from build123d import *

# Parameters (mm, degrees)
CUT_EXTRUDE_1_DEPTH = 0.495


with BuildPart() as part:
    # 草图1 → 旋转1 (revolve)
    with BuildSketch(Plane.XY, mode=Mode.PRIVATE) as revolve_1_sk:
        with BuildLine():
            Line((0, 0), (2.75, 0))
            Line((2.75, 0), (1.747011561, 1.038624933))
            ThreePointArc((1.747011561, 1.038624933), (1.564086143, 1.320305375), (1.5, 1.65))
            Line((1.5, 1.65), (1.5, 10))
            Line((1.5, 10), (0, 10))
            Line((0, 10), (0, 0))
        make_face()
    revolve(revolve_1_sk.sketch.rotate(Axis((0, 3.09547163, 0), (0, -1, 0)), 90), axis=Axis((0, 3.09547163, 0), (0, -1, 0)))

    # 草图2 → 切除-拉伸1 (cut)
    with BuildSketch(Plane.XZ):
        Polygon((-0.375, -0.375), (-0.375, -1.925), (0.375, -1.925), (0.375, -0.375), (1.925, -0.375), (1.925, 0.375), (0.375, 0.375), (0.375, 1.925), (-0.375, 1.925), (-0.375, 0.375), (-1.925, 0.375), (-1.925, -0.375), align=None)
    extrude(amount=-CUT_EXTRUDE_1_DEPTH, mode=Mode.SUBTRACT)


solid = part.part
For this review, take the finished solid that the model builds, in its own axes (mm). Round coordinates to 2 decimals unless told otherwise and drop trailing zeros. Order: outer loops, then holes, each group sorted by start corner. A loop starts at its lowest first (then second) coordinate and runs counter-clockwise, first axis right, second up. Notation, with made-up numbers: M 31,67 L 49,67 A29 cw 49,100 Z; hole C -2.75,39 d7. An arc over 180 degrees is marked long. Write each question's results on one line, items separated by ' | '. Start each with the question number.
1. Add section B-B (x = 0). State the section outline as (y, z) points (3 decimals), then the cut area to 3 significant figures.
2. Add section C-C (y = 7.5). State the section outline as (x, z) points, then the cut area to 3 significant figures.
3. Clearance check with flat-ended pins moving along their axes: pin 1 Ø3 at (x, y) = (0, 8.5) entering from -Z; pin 2 Ø0.5 at (y, z) = (0, -1.5) entering from +X. State where each tip first meets the part, or that it passes through.
4. To check wall thickness, follow L1, parallel to Y at x = 1.45, z = -0.15 (3 decimals); L2, parallel to X at y = 6.75, z = -0.15; L3, parallel to X at y = 5, z = -1.3. State the ranges of each line that lie inside material, in increasing order. Write a range as [from, to].
5. Draft analysis for pull direction X (two halves, no side actions). For faces 1 (the face through (-0.45, 5.88, 1.43)), 2 (the face through (0, 0.495, 0)), 3 (the face through (1, 0, -1)), state which applies: pulls with the +X half, pulls with the -X half, needs draft (parallel to the pull), parting line crosses it, or undercut.
6. Add section A-A (z = 0). State the section outline as (x, y) points (3 decimals), then the cut area to 3 significant figures.
Output values:
1) outline: M 0,-2.75 L 1.039,-1.747 A0.88 cw 1.65,-1.5 L 10,-1.5 L 10,1.5 L 1.65,1.5 A0.88 cw 1.039,1.747 L 0,2.75 L 0,1.925 L 0.495,1.925 L 0.495,-1.925 L 0,-1.925 Z | area: 29.7 mm^2
2) outline: C 0,0 d3 | area: 7.07 mm^2
3) pin 1: z = -1.5 | pin 2: x = 2.45
4) L1: [0.495, 10] | L2: [-1.49, 1.49] | L3: [-0.75, 0.75]
5) face 1: parting line crosses it | face 2: undercut | face 3: needs draft
6) outline: M -2.75,0 L -1.925,0 L -1.925,0.495 L 1.925,0.495 L 1.925,0 L 2.75,0 L 1.747,1.039 A0.88 cw 1.5,1.65 L 1.5,10 L -1.5,10 L -1.5,1.65 A0.88 cw -1.747,1.039 Z | area: 29.7 mm^2
